Model file for the job. Use its own axes, mm. A direction names the side the tool comes from. Round coordinates to 2 decimals unless told otherwise and drop trailing zeros. Loops run counter-clockwise (first coordinate to the right, second up) from the corner with the lowest first, then second, coordinate; pieces in that order, holes last. Notation, with made-up numbers: (-7.5, -15.5) - (2.5, -15.5) arc R11 cw to (2.5, -11.5) - close; hole circle Ø4 at (45.25, 46). An arc over 180 degrees is marked (long way). Use one line per item in the form item = value.
from build123d import *

# Parameters (mm, degrees)
SKETCH1_W                = 200
SKETCH1_H                = 213
BOSS_EXTRUDE1_DEPTH      = 25
FILLET1_R                = 10
BOSS_EXTRUDE2_START      = 10
BOSS_EXTRUDE2_DEPTH      = 10
BOSS_EXTRUDE3_DEPTH      = 95
BOSS_EXTRUDE4_DEPTH      = 10
BOSS_EXTRUDE4_DEPTH_BACK = 120
SKETCH4_R                = 35
CUT_EXTRUDE1_DEPTH       = 290.575983208
CUT_EXTRUDE1_DEPTH_BACK  = 290.575983208
SKETCH6_R                = 20.5
BOSS_EXTRUDE5_DEPTH      = 10
BOSS_EXTRUDE5_DEPTH_BACK = 120
SKETCH7_R                = 41.5
CUT_EXTRUDE2_DEPTH       = 290.766716644
CUT_EXTRUDE2_DEPTH_BACK  = 290.766716644
SKETCH8_R                = 20.5
CHAMFER1_SIZE            = 4
CUT_EXTRUDE3_DEPTH       = 10
SKETCH10_R               = 13.920178612
CUT_EXTRUDE4_DEPTH       = 10
SKETCH11_R               = 8.357374053
CUT_EXTRUDE5_DEPTH       = 211.486341717


with BuildPart() as part:
    # Sketch1 → Boss-Extrude1 (new body)
    with BuildSketch(Plane(origin=(0, 0, 0), x_dir=(1, 0, 0), z_dir=(0, 1, 0))):
        Rectangle(SKETCH1_W, SKETCH1_H)
    extrude(amount=BOSS_EXTRUDE1_DEPTH)

    # Fillet1
    fillet1_edges = [part.edges().sort_by_distance(p)[0] for p in [
        (100, 12.5, 106.5),
        (-100, 12.5, 106.5),
        (-100, 12.5, -106.5),
        (100, 12.5, -106.5),
    ]]
    fillet(fillet1_edges, radius=FILLET1_R)

    # Sketch2 → Boss-Extrude2 (add)
    with BuildSketch(Plane(origin=(0, 25, 0), x_dir=(1, 0, 0), z_dir=(0, 1, 0)).offset(BOSS_EXTRUDE2_START)):
        with BuildLine():
            Line((50, -46.5), (100, -46.5))
            Line((100, -46.5), (100, -96.5))
            ThreePointArc((100, -96.5), (97.071067812, -103.571067812), (90, -106.5))
            Line((90, -106.5), (40, -106.5))
            Line((40, -106.5), (40, -56.5))
            ThreePointArc((40, -56.5), (42.928932188, -49.428932188), (50, -46.5))
        make_face()
    extrude(amount=-BOSS_EXTRUDE2_DEPTH)

    # Sketch3 → Boss-Extrude3 (add)
    with BuildSketch(Plane(origin=(0, 25, 0), x_dir=(1, 0, 0), z_dir=(0, 1, 0))):
        with BuildLine():
            Line((100, 63.5), (20, 63.5))
            ThreePointArc((20, 63.5), (-6.360389693, -0.139610307), (-70, -26.5))
            Line((-70, -26.5), (-70, -106.5))
            Line((-70, -106.5), (-61, -106.5))
            Line((-61, -106.5), (-61, -35.090060351))
            ThreePointArc((-61, -35.090060351), (0.003571337, -6.503571337), (28.590060351, 54.5))
            Line((28.590060351, 54.5), (100, 54.5))
            Line((100, 54.5), (100, 63.5))
        make_face()
    extrude(amount=BOSS_EXTRUDE3_DEPTH)

    # Sketch4 → Boss-Extrude4 (add, two sides: drawn at the far end of the back side and taken through both)
    with BuildSketch(Plane.XY.offset(106.5).offset(-BOSS_EXTRUDE4_DEPTH_BACK)):
        with Locations((-65.5, 120)):
            Circle(SKETCH4_R)
    extrude(amount=BOSS_EXTRUDE4_DEPTH + BOSS_EXTRUDE4_DEPTH_BACK)

    # Sketch6 → Cut-Extrude1 (cut, two sides: drawn at the far end of the back side and taken through both)
    with BuildSketch(Plane.XY.offset(116.5).offset(-CUT_EXTRUDE1_DEPTH_BACK)):
        with Locations((-65.5, 120)):
            Circle(SKETCH6_R)
    extrude(amount=CUT_EXTRUDE1_DEPTH + CUT_EXTRUDE1_DEPTH_BACK, mode=Mode.SUBTRACT)

    # Sketch7 → Boss-Extrude5 (add, two sides: drawn at the far end of the back side and taken through both)
    with BuildSketch(Plane(origin=(100, 0, 0), x_dir=(0, 0, -1), z_dir=(1, 0, 0)).offset(-BOSS_EXTRUDE5_DEPTH_BACK)):
        with Locations((59, 120)):
            Circle(SKETCH7_R)
    extrude(amount=BOSS_EXTRUDE5_DEPTH + BOSS_EXTRUDE5_DEPTH_BACK)

    # Sketch8 → Cut-Extrude2 (cut, two sides: drawn at the far end of the back side and taken through both)
    with BuildSketch(Plane(origin=(110, 0, 0), x_dir=(0, 0, -1), z_dir=(1, 0, 0)).offset(-CUT_EXTRUDE2_DEPTH_BACK)):
        with Locations((59, 120)):
            Circle(SKETCH8_R)
    extrude(amount=CUT_EXTRUDE2_DEPTH + CUT_EXTRUDE2_DEPTH_BACK, mode=Mode.SUBTRACT)

    # Chamfer1
    chamfer1_edges = [part.edges().sort_by_distance(p)[0] for p in [
        (-20, 120, -38.5),
        (110, 120, -38.5),
        (-86, 120, -13.5),
        (-86, 120, 116.5),
    ]]
    chamfer(chamfer1_edges, length=CHAMFER1_SIZE)

    # Sketch9 → Cut-Extrude3 (cut)
    with BuildSketch(Plane(origin=(0, 25, 0), x_dir=(1, 0, 0), z_dir=(0, 1, 0))):
        with BuildLine():
            Line((81, 45.5), (44.629839047, 45.5))
            ThreePointArc((44.629839047, 45.5), (38.454436775, 43.365392983), (34.915445908, 37.872881356))
            ThreePointArc((34.915445908, 37.872881356), (6.367532368, -12.867532368), (-44.372881356, -41.415445908))
            ThreePointArc((-44.372881356, -41.415445908), (-49.865392983, -44.954436775), (-52, -51.129839047))
            Line((-52, -51.129839047), (-52, -87.5))
            ThreePointArc((-52, -87.5), (-49.071067812, -94.571067812), (-42, -97.5))
            Line((-42, -97.5), (21, -97.5))
            ThreePointArc((21, -97.5), (28.071067812, -94.571067812), (31, -87.5))
            Line((31, -87.5), (31, -56.5))
            ThreePointArc((31, -56.5), (36.564971157, -43.064971157), (50, -37.5))
            Line((50, -37.5), (81, -37.5))
            ThreePointArc((81, -37.5), (88.071067812, -34.571067812), (91, -27.5))
            Line((91, -27.5), (91, 35.5))
            ThreePointArc((91, 35.5), (88.071067812, 42.571067812), (81, 45.5))
        make_face()
    extrude(amount=-CUT_EXTRUDE3_DEPTH, mode=Mode.SUBTRACT)

    # Sketch10 → Cut-Extrude4 (cut)
    with BuildSketch(Plane(origin=(0, 35, 0), x_dir=(1, 0, 0), z_dir=(0, 1, 0))):
        with Locations(Location((70, -76.5, 0), (0, 0, 270))):
            Circle(SKETCH10_R)
    extrude(amount=-CUT_EXTRUDE4_DEPTH, mode=Mode.SUBTRACT)

    # Sketch11 → Cut-Extrude5 (cut, through all)
    with BuildSketch(Plane(origin=(0, 25, 0), x_dir=(1, 0, 0), z_dir=(0, 1, 0))):
        with Locations(Location((70, -76.5, 0), (0, 0, 270))):
            Circle(SKETCH11_R)
    extrude(amount=-CUT_EXTRUDE5_DEPTH, mode=Mode.SUBTRACT)


solid = part.part
1. Wall check: probe 1 along Y at (x, z) = (-64.5, 9.5); probe 2 along Y at (x, z) = (17.5, -59); probe 3 along X at (y, z) = (29, 76.5). Give the ranges that are in metal, low to high.
Geometry check:
probe_1 = 0 to 25, 85.01 to 99.52, 140.48 to 154.99
probe_2 = 0 to 25, 78.5 to 99.5, 140.5 to 161.5
probe_3 = -70 to -61, 40 to 56.08, 83.92 to 100
2. Cut at B-B, the plane z = -59. Give the cut face in (x, y), plus the area to 3 significant figures.
Geometry check:
outline = (-100, 0) - (100, 0) - (100, 78.5) - (110, 78.5) - (110, 95.5) - (106, 99.5) - (-16, 99.5) - (-20, 95.5) - (-20, 78.5) - (19.89, 78.5) - (19.89, 25) - (-100, 25) - close; (-20, 144.5) - (-16, 140.5) - (106, 140.5) - (110, 144.5) - (110, 161.5) - (-20, 161.5) - close
area = 14,700 mm^2
3. Cut at D-D, the plane x = 13. Give the cut face in (y, z).
Geometry check:
outline = (0, -106.5) - (25, -106.5) - (25, -28.7) - (91.64, -28.7) arc R41.5 ccw (long way) to (120, -17.5) - (120, -9.54) - (25, -9.54) - (25, 5.6) - (15, 5.6) - (15, 97.5) - (25, 97.5) - (25, 106.5) - (0, 106.5) - close; hole circle Ø41 at (120, -59)
4. Flat gauge pins, fed straight in: pin 1 (6 mm diameter, centred on x = -48.5, z = -62, fed in from +Y); pin 2 (25 mm diameter, centred on y = 103.5, z = -62, fed in from -X); pin 3 (2 mm diameter, centred on x = -10, y = 28.5, fed in from -Z). Where does each tip first touch, or does it go through?
Geometry check:
pin_1 = 25
pin_2 = -20
pin_3 = 2.67
5. Cut at C-C, the plane x = -65.5. Give the cut face in (y, z).
Geometry check:
outline = (0, -106.5) - (25, -106.5) - (25, 26.39) - (85, 26.39) - (85, -13.5) - (95.5, -13.5) - (99.5, -9.5) - (99.5, 112.5) - (95.5, 116.5) - (85, 116.5) - (85, 106.5) - (0, 106.5) - close; (140.5, -9.5) - (144.5, -13.5) - (155, -13.5) - (155, 116.5) - (144.5, 116.5) - (140.5, 112.5) - close
6. Pull direction Z, two halves, no side cores. Call faces 6 (the cylindrical face through (-5.664, 61.279, -0.564)), 7 (the flat face through (-24, 25, -49)), 8 (the cylindrical face through (-49.808, 20.07, 44.881)), 9 (the flat face through (-1, 12, -106.5)): +Z half, -Z half, draft (parallel to the pull), parting line (faces both ways), or undercut.
Geometry check:
face_6 = undercut
face_7 = draft
face_8 = undercut
face_9 = -Z half
7. Tool access for faces 1 (the flat face through (40, 30, 82)), 2 (the flat face through (-7, 120, 5)), 3 (the cylindrical face through (-97.15, 12.68, 103.49)), 4 (the flat face through (64, 51, -54.5)), 5 (the cylindrical face through (42.85, 30.07, 49.51)): list every direction of +Z, -Z, +X, -X, +Y, -Y with a clear straight run to the whole face (end or side of a thin tool).
Geometry check:
face_1 = +Z, +Y
face_2 = +Z, +X, +Y
face_3 = +Z, -X, -Y
face_4 = +X
face_5 = +Y
8. Cut at A-A, the plane x = 70. Give the cut face in (y, z).
Geometry check:
outline = (0, -106.5) - (25, -106.5) - (25, -63.5) - (78.74, -63.5) arc R41.5 ccw (long way) to (78.74, -54.5) - (25, -54.5) - (25, -45.5) - (15, -45.5) - (15, 37.5) - (25, 37.5) - (25, 46.5) - (35, 46.5) - (35, 62.58) - (25, 62.58) - (25, 68.14) - (0, 68.14) - close; (0, 84.86) - (25, 84.86) - (25, 90.42) - (35, 90.42) - (35, 106.5) - (0, 106.5) - close; hole circle Ø41 at (120, -59)
